Geometry check sheet. Reference: the model listing, model coordinates, mm. A direction names the side the tool comes from. Round coordinates to 2 decimals unless told otherwise and drop trailing zeros. Loops run counter-clockwise (first coordinate to the right, second up) from the corner with the lowest first, then second, coordinate; pieces in that order, holes last. Notation, with made-up numbers: (-18.5, 11) - (24.5, 11) arc R25 ccw to (24.5, 26) - close; hole circle Ø10 at (54.25, 12). An arc over 180 degrees is marked (long way). Answer in a Markdown table with one row per item. Add a question column.
```python
from build123d import *

# Parameters (mm, degrees)
SKETCH1_W           = 63.5
SKETCH1_H           = 76.2
BOSS_EXTRUDE1_DEPTH = 12.7
SKETCH2_W           = 63.5
SKETCH2_H           = 51.435
CUT_EXTRUDE1_DEPTH  = 5.08
SKETCH3_R           = 14.605
CUT_EXTRUDE2_DEPTH  = 7.62
SKETCH4_R           = 3.4925
CUT_EXTRUDE4_DEPTH  = 12.7
SKETCH6_R           = 17.145
CUT_EXTRUDE6_DEPTH  = 2.54


with BuildPart() as part:
    # Sketch1 → Boss-Extrude1 (new body)
    with BuildSketch(Plane(origin=(0, 0, 0), x_dir=(1, 0, 0), z_dir=(0, 1, 0))):
        with Locations((31.75, -38.1)):
            Rectangle(SKETCH1_W, SKETCH1_H)
    extrude(amount=BOSS_EXTRUDE1_DEPTH)

    # Sketch2 → Cut-Extrude1 (cut)
    with BuildSketch(Plane(origin=(0, 12.7, 0), x_dir=(1, 0, 0), z_dir=(0, 1, 0))):
        with Locations((31.75, -38.1)):
            Rectangle(SKETCH2_W, SKETCH2_H)
    extrude(amount=-CUT_EXTRUDE1_DEPTH, mode=Mode.SUBTRACT)

    # Sketch3 → Cut-Extrude2 (cut)
    with BuildSketch(Plane(origin=(0, 7.62, 0), x_dir=(1, 0, 0), z_dir=(0, 1, 0))):
        with Locations(Location((31.75, -38.1, 0), (0, 0, 270))):
            Circle(SKETCH3_R)
    extrude(amount=-CUT_EXTRUDE2_DEPTH, mode=Mode.SUBTRACT)

    # Sketch4 → Cut-Extrude4 (cut)
    with BuildSketch(Plane(origin=(0, 12.7, 0), x_dir=(1, 0, 0), z_dir=(0, 1, 0))):
        with Locations(Location((7.62, -6.19125, 0), (0, 0, 270))):
            Circle(SKETCH4_R)
        with Locations(Location((55.88, -6.19125, 0), (0, 0, 270))):
            Circle(SKETCH4_R)
        with Locations(Location((7.62, -70.00875, 0), (0, 0, 270))):
            Circle(SKETCH4_R)
        with Locations(Location((55.88, -70.00875, 0), (0, 0, 270))):
            Circle(SKETCH4_R)
    extrude(amount=-CUT_EXTRUDE4_DEPTH, mode=Mode.SUBTRACT)

    # Sketch6 → Cut-Extrude6 (cut)
    with BuildSketch(Plane(origin=(0, 7.62, 0), x_dir=(1, 0, 0), z_dir=(0, 1, 0))):
        with Locations(Location((31.75, -38.1, 0), (0, 0, 270))):
            Circle(SKETCH6_R)
    extrude(amount=-CUT_EXTRUDE6_DEPTH, mode=Mode.SUBTRACT)


solid = part.part
```
Q1. Cross-section at D-D, the plane y = 6. State how many separate pieces and enclosed holes the cut face has, plus the area to 3 significant figures.
Q2. Cross-section at B-B, the plane z = 38.1. Enter the section's corners in (x, y) (3 decimals), plus the area to 3 significant figures.
Q3. Cross-section at A-A, the plane x = 55.88. Enter the section's corners in (y, z), plus the area to 3 significant figures.
Q4. Cross-section at C-C, the plane x = 31.75. Enter the section's corners in (y, z) (1 decimal), plus the area to 3 significant figures.
Q5. Set-up check for faces 5 (the flat face through (45, 0, 29)), 6 (the flat face through (31, 10, 63.818)), 7 (the flat face through (39, 5.08, 51)): record each of +Z, -Z, +X, -X, +Y, -Y from which the full face is reachable in a straight line by a thin tool's end or side.
Q6. Scan lines: line 1 (Z direction, x = 7.5, y = 1.75); line 2 (Z direction, x = 55, y = 10.25); line 3 (X direction, y = 7.5, z = 73). Record each from-to range of solid material in increasing order. Write a range as from..to.
Q7. Release check for a two-part mould opening along X. For faces 1 (the cylindrical face through (54.542, 6.439, 73.235)), 2 (the cylindrical face through (11.083, 6.439, 5.737)), 3 (the flat face through (63.5, 5, 39)), 4 (the flat face through (31, 10, 12.382)) record: +X half, -X half, draft (parallel to the pull), parting line (faces both ways), or undercut.
Q8. Depth check by flat-ended pin: P1, Ø6.5, axis at x = 7.62, z = 6.19, coming from the -Y side; P2, Ø9, axis at x = 7.62, z = 70.01, coming from the -Y side; P3, Ø6, axis at x = 10.5, z = 44.5, coming from the +Y side. Enter the tip coordinate at first touch or a pass-through.
Check sheet entries:
| question | item | result |
|---|---|---|
| 1 | separate pieces | 1 |
| 1 | enclosed holes | 5 |
| 1 | area | 3,760 mm² |
| 2 | outline | (0, 0) - (17.145, 0) - (17.145, 5.08) - (14.605, 5.08) - (14.605, 7.62) - (0, 7.62) - close; (46.355, 0) - (63.5, 0) - (63.5, 7.62) - (48.895, 7.62) - (48.895, 5.08) - (46.355, 5.08) - close |
| 2 | area | 248 mm² |
| 3 | outline | (0, 0) - (12.7, 0) - (12.7, 2.7) - (0, 2.7) - close; (0, 9.68) - (12.7, 9.68) - (12.7, 12.38) - (7.62, 12.38) - (7.62, 63.82) - (12.7, 63.82) - (12.7, 66.52) - (0, 66.52) - close; (0, 73.5) - (12.7, 73.5) - (12.7, 76.2) - (0, 76.2) - close |
| 3 | area | 529 mm² |
| 4 | outline | (0, 0) - (12.7, 0) - (12.7, 12.4) - (7.6, 12.4) - (7.6, 21) - (5.1, 21) - (5.1, 23.5) - (0, 23.5) - close; (0, 52.7) - (5.1, 52.7) - (5.1, 55.2) - (7.6, 55.2) - (7.6, 63.8) - (12.7, 63.8) - (12.7, 76.2) - (0, 76.2) - close |
| 4 | area | 471 mm² |
| 5 | face 5 | +Z, -Z, +X, -X, -Y |
| 5 | face 6 | +X, -X, +Y |
| 5 | face 7 | +Y |
| 6 | line 1 | 0..2.7, 9.68..66.52, 73.5..76.2 |
| 6 | line 2 | 0..2.81, 9.57..12.38, 63.82..66.63, 73.39..76.2 |
| 6 | line 3 | 0..5.82, 9.42..54.08, 57.68..63.5 |
| 7 | face 1 | undercut |
| 7 | face 2 | undercut |
| 7 | face 3 | +X half |
| 7 | face 4 | draft |
| 8 | P1 | through |
| 8 | P2 | y = 0 |
| 8 | P3 | y = 7.62 |
